Source: CAD feature listing. Evaluate the final solid. Frame: model axes, mm. Give positions to 0.01 mm unless a question says otherwise; leave off trailing zeros. Order: outer loops, then holes, each group sorted by start corner. A loop starts at its lowest first (then second) coordinate and runs counter-clockwise, first axis right, second up. Notation, with made-up numbers: M -26.5,-11.5 L -18.5,-11.5 A9 ccw -18.5,2.5 Z; hole C 74.5,36.25 d2. An arc over 180 degrees is marked long. Return JSON: item names as keys, results as strings.
Solid Edge part; units mm, degrees
sketch "Sketch1" plane through (0, 0, 0) normal (0, 0, 1) x (1, 0, 0)
  line L0 (-12.7, -101.6) -> (12.7, -101.6)
  line L1 (12.7, -101.6) -> (12.7, 101.6)
  line L2 (12.7, 101.6) -> (-12.7, 101.6)
  line L3 (-12.7, 101.6) -> (-12.7, -101.6)
  dimension "D1" = 12.7
  dimension "D2" = 12.7
extrude "Protrusion1" add sketch "Sketch1" along normal blind 6.35
hole "Hole_1" at (0, 88.9, 6.35) direction (0, 0, -1) diameter 6.35 end up to next
fillet "Round_1" radius 3.175 4 edges at (12.7, 101.6, 3.175) (-12.7, 101.6, 3.175) (12.7, -101.6, 3.175) (-12.7, -101.6, 3.175)
properties part number "SPaRC 02 - 004"
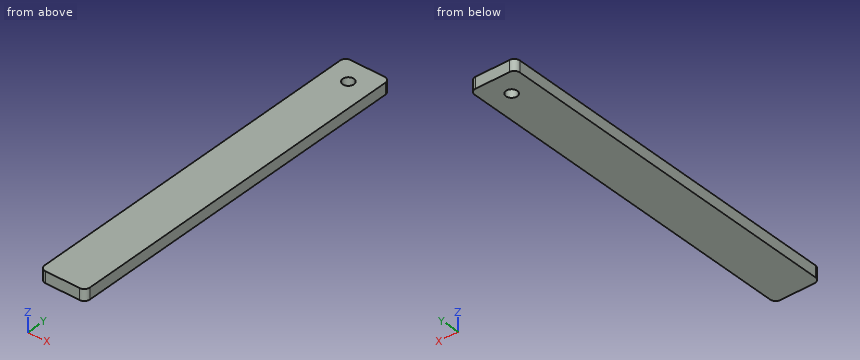
1. Ray query, probe 1 along X at (y, z) = (88.9, 2) (3 decimals); probe 2 along Y at (x, z) = (0, 4.5) (3 decimals); probe 3 along X at (y, z) = (88, 4). Return the intervals inside material, ascending.
Evaluation:
{"probe 1": "x = -12.7 to -3.175, 3.175 to 12.7", "probe 2": "y = -101.6 to 85.725, 92.075 to 101.6", "probe 3": "x = -12.7 to -3.04, 3.04 to 12.7"}
2. Section query B-B (y = 88.9). Return loops of the section in (x, z) (3 decimals).
Evaluation:
{"outline": "M -12.7,0 L -3.175,0 L -3.175,6.35 L -12.7,6.35 Z; M 3.175,0 L 12.7,0 L 12.7,6.35 L 3.175,6.35 Z"}
3. First-contact query: pin 1 (5 mm diameter, centred on x = 5, y = -68, fed in from -Z). Flat tip, straight axial feed; report the tip coordinate or a pass-through.
Evaluation:
{"pin 1": "stops at z = 0"}
4. Section query A-A (x = 0). Return loops of the section in (y, z) (3 decimals).
Evaluation:
{"outline": "M -101.6,0 L 85.725,0 L 85.725,6.35 L -101.6,6.35 Z; M 92.075,0 L 101.6,0 L 101.6,6.35 L 92.075,6.35 Z"}
